For this review, take the finished solid that the model builds, in its own axes (mm). Coordinates: 2 decimals unless noted, no trailing zeros. Loops run counter-clockwise (first coordinate to the right, second up) from the corner with the lowest first, then second, coordinate; pieces in that order, holes last. Notation, with made-up numbers: (-15.75, 60) -> (-0.75, 60) arc R22 ccw to (-0.75, 77) -> close; hole circle Ø8 at (3.25, 63). An arc over 180 degrees is marked (long way). Use a Markdown table: item, result.
Autodesk Fusion 360 part; units mm, degrees
sketch "Sketch1" plane through (0, 0, 0) normal (0, 0, 1) x (1, 0, 0)
  circle A0 centre (0, 0) radius 12
  circle A1 centre (0, 0) radius 22.5
  circle A2 centre (0, 0) radius 38
  dimension "d1" = 45
  dimension "d2" = 24
  dimension "d3" = 76
extrude "Extrude1" add sketch "Sketch1" along normal blind 20 contours A1
sketch "Sketch2" plane through (0, 0, 0) normal (0, 0, 1) x (1, 0, 0)
  circle A0 centre (0.2654, -30.1553) radius 2.5
  dimension "d8" = 5
extrude "Extrude4" add sketch "Sketch1" along normal blind 2 contours A1 | A2
extrude "Extrude5" cut sketch "Sketch2" along normal blind 6.312
pattern_circular "C-Pattern2" count 3 over 360 about axis through (0, 0, 2) along (0, 0, 1) of "Extrude5"
extrude "돌출6" add 1 faces at (-20.8034, 21.3677, 2) along direction (0, 0, 1) blind 18
(1) For pin 1 Ø1.5 at (x, z) = (-16, 9) entering from -Y; pin 2 Ø4 at (x, y) = (-26.25, 14.85) entering from +Z; pin 3 Ø2 at (x, y) = (26.5, -23) entering from -Z; pin 4 Ø2 at (y, z) = (-25.5, 4) entering from +X, all flat-tipped, find the tip position at first contact; note any pin that passes through.
Found:
| item | result |
|---|---|
| pin 1 | stops at y = -34.81 |
| pin 2 | passes through |
| pin 3 | stops at z = 0 |
| pin 4 | stops at x = 29.05 |
(2) Take a section at B-B on x = -3.5. Write out the cut boundary in (y, z), plus the area to 3 significant figures.
Found:
| item | result |
|---|---|
| outline | (-37.84, 0) -> (-11.48, 0) -> (-11.48, 20) -> (-37.84, 20) -> close; (11.48, 0) -> (37.84, 0) -> (37.84, 20) -> (11.48, 20) -> close |
| area | 1,050 mm^2 |
(3) For line 1 along X through (y, z) = (-9.5, 13); line 2 along X through (y, z) = (-29.5, 12.5); line 3 along Y through (x, z) = (-10.5, 13.5), list the stretches that pass through material, from the lowest coordinate up.
Found:
| item | result |
|---|---|
| line 1 | x = -36.79 to -7.33, 7.33 to 36.79 |
| line 2 | x = -23.95 to -2.15, 2.68 to 23.95 |
| line 3 | y = -36.52 to -5.81, 5.81 to 36.52 |
(4) Mouldability with a two-part tool opening along Y and no side actions: class faces 1 (the face through (-23.863, 14.097, 9.86)), 2 (the face through (17.535, 33.713, 9.86)), 3 (the face through (-9, 9, 0)) as pulls with the +Y half, pulls with the -Y half, needs draft (parallel to the pull), parting line crosses it, or undercut.
Found:
| item | result |
|---|---|
| face 1 | undercut |
| face 2 | parting line crosses it |
| face 3 | needs draft |
(5) Take a section at A-A on y = 0. Write out the cut boundary in (x, z), plus the area to 3 significant figures.
Found:
| item | result |
|---|---|
| outline | (-38, 0) -> (-12, 0) -> (-12, 20) -> (-38, 20) -> close; (12, 0) -> (38, 0) -> (38, 20) -> (12, 20) -> close |
| area | 1,040 mm^2 |
(6) Take a section at C-C on z = 6. Write out the cut boundary in (x, y).
Found:
| item | result |
|---|---|
| outline | circle Ø76 at (0, 0); hole circle Ø5 at (-26.25, 14.85); hole circle Ø24 at (0, 0); hole circle Ø5 at (0.27, -30.16); hole circle Ø5 at (25.98, 15.31) |
(7) Take a section at D-D on y = -17. Write out the cut boundary in (x, z), plus the area to 3 significant figures.
Found:
| item | result |
|---|---|
| outline | (-33.99, 0) -> (33.99, 0) -> (33.99, 20) -> (-33.99, 20) -> close |
| area | 1,360 mm^2 |
